```python
from build123d import *

# Parameters (mm, degrees)
SKETCH1_R                          = 14
BOSS_EXTRUDE1_DEPTH                = 20.5
SKETCH2_R                          = 12
CUT_EXTRUDE1_DEPTH                 = 17.5
CHAMFER1_SIZE                      = 1.5
SKETCH3_W                          = 0.15
SKETCH3_H                          = 0.25
SKETCH4_R                          = 4.45
BOSS_EXTRUDE2_DEPTH                = 1.5
BOSS_EXTRUDE2_DEPTH_BACK           = 4.5
SKETCH10_R                         = 4.45
BOSS_EXTRUDE3_DEPTH                = 3.5
BOSS_EXTRUDE3_TAPER                = 30
SKETCH5_R                          = 1.5
CUT_EXTRUDE2_DEPTH                 = 23
CUT_EXTRUDE3_DEPTH                 = 4.5
M1_6X0_35_TAPPED_HOLE1_D           = 1.25
M1_6X0_35_TAPPED_HOLE1_DEPTH       = 4.25
M1_6X0_35_TAPPED_HOLE1_TIP         = 0.375537887
M2_CLEARANCE_HOLE4_D               = 2.2
M2_CLEARANCE_HOLE4_DEPTH           = 3.5
M2_CLEARANCE_HOLE4_TIP             = 0.660946681
M2_CLEARANCE_HOLE4_ON_FACE_2_D     = 2.2
M2_CLEARANCE_HOLE4_ON_FACE_2_DEPTH = 3.5
M2_CLEARANCE_HOLE4_ON_FACE_2_TIP   = 0.660946681


with BuildPart() as part:
    # Sketch1 → Boss-Extrude1 (new body)
    with BuildSketch(Plane(origin=(0, 0, 0), x_dir=(1, 0, 0), z_dir=(0, 1, 0))):
        Circle(SKETCH1_R)
    extrude(amount=BOSS_EXTRUDE1_DEPTH)

    # Sketch2 → Cut-Extrude1 (cut)
    with BuildSketch(Plane.XZ):
        Circle(SKETCH2_R)
    extrude(amount=-CUT_EXTRUDE1_DEPTH, mode=Mode.SUBTRACT)

    # Chamfer1
    chamfer1_edges = [part.edges().sort_by_distance(p)[0] for p in [
        (-14, 20.5, 0),
    ]]
    chamfer(chamfer1_edges, length=CHAMFER1_SIZE)

    # Sketch3 → Cut-Revolve1 (revolve, cut)
    with BuildSketch(Plane(origin=(0, 0, 0), x_dir=(0, 0, -1), z_dir=(1, 0, 0))):
        with Locations((13.925, 14.875)):
            Rectangle(SKETCH3_W, SKETCH3_H)
    revolve(axis=Axis((0, 20.5, 0), (0, -1, 0)), mode=Mode.SUBTRACT)

    # Sketch4 → Boss-Extrude2 (add, two sides)
    with BuildSketch(Plane(origin=(0, 20.5, 0), x_dir=(1, 0, 0), z_dir=(0, 1, 0))) as boss_extrude2_sk:
        Circle(SKETCH4_R)
    extrude(amount=BOSS_EXTRUDE2_DEPTH)
    extrude(boss_extrude2_sk.sketch, amount=-BOSS_EXTRUDE2_DEPTH_BACK)

    # Sketch10 → Boss-Extrude3 (add)
    with BuildSketch(Plane.XZ.offset(-16)):
        Circle(SKETCH10_R)
    extrude(amount=BOSS_EXTRUDE3_DEPTH, taper=BOSS_EXTRUDE3_TAPER)

    # Sketch5 → Cut-Extrude2 (cut, through all)
    with BuildSketch(Plane(origin=(0, 22, 0), x_dir=(1, 0, 0), z_dir=(0, 1, 0))):
        Circle(SKETCH5_R)
    extrude(amount=-CUT_EXTRUDE2_DEPTH, mode=Mode.SUBTRACT)

    # Sketch6 → Cut-Extrude3 (cut)
    with BuildSketch(Plane(origin=(0, 20.5, 0), x_dir=(1, 0, 0), z_dir=(0, 1, 0))):
        with BuildLine():
            ThreePointArc((-10.0036, -7.495197598), (-4.6, 0), (-10.0036, 7.495197598))
            ThreePointArc((-10.0036, 7.495197598), (-12.5, 0), (-10.0036, -7.495197598))
        make_face()
        with BuildLine():
            ThreePointArc((-10.0036, 7.495197598), (-10.789488556, 7.712596878), (-11.5936, 7.847830212))
            ThreePointArc((-11.5936, 7.847830212), (-14, 0), (-11.5936, -7.847830212))
            ThreePointArc((-11.5936, -7.847830212), (-10.789488556, -7.712596878), (-10.0036, -7.495197598))
            ThreePointArc((-10.0036, -7.495197598), (-12.5, 0), (-10.0036, 7.495197598))
        make_face()
        with BuildLine():
            ThreePointArc((-9.006237245, -8.668199968), (-6.25, -10.825317547), (-3.003762755, -12.133730231))
            ThreePointArc((-3.003762755, -12.133730231), (-4.5, -7.794228634), (-9.006237245, -8.668199968))
        make_face()
        with BuildLine():
            ThreePointArc((-9.677498914, -10.116620719), (-7, -12.124355653), (-3.922501086, -13.439270264))
            ThreePointArc((-3.922501086, -13.439270264), (-3.387703302, -12.839581088), (-3.003762755, -12.133730231))
            ThreePointArc((-3.003762755, -12.133730231), (-6.25, -10.825317547), (-9.006237245, -8.668199968))
            ThreePointArc((-9.006237245, -8.668199968), (-9.425551745, -9.353627664), (-9.677498914, -10.116620719))
        make_face()
        with BuildLine():
            ThreePointArc((-0.999620328, -13.964267227), (7, -12.124355653), (12.593220328, -6.116437015))
            ThreePointArc((12.593220328, -6.116437015), (12.074049103, -5.487672744), (11.492831527, -4.91577293))
            ThreePointArc((11.492831527, -4.91577293), (6.25, -10.825317547), (-1.489231527, -12.410970529))
            ThreePointArc((-1.489231527, -12.410970529), (-1.284560547, -13.200269622), (-0.999620328, -13.964267227))
        make_face()
        with BuildLine():
            ThreePointArc((-1.489231527, -12.410970529), (6.25, -10.825317547), (11.492831527, -4.91577293))
            ThreePointArc((11.492831527, -4.91577293), (2.3, -3.983716857), (-1.489231527, -12.410970529))
        make_face()
        with BuildLine():
            ThreePointArc((12.5, 0), (12.376893794, 1.75), (12.01, 3.465530262))
            ThreePointArc((12.01, 3.465530262), (9, 0), (12.01, -3.465530262))
            ThreePointArc((12.01, -3.465530262), (12.376893794, -1.75), (12.5, 0))
        make_face()
        with BuildLine():
            ThreePointArc((13.6, -3.322649545), (13.899640283, -1.673320053), (14, 0))
            ThreePointArc((14, 0), (13.899640283, 1.673320053), (13.6, 3.322649545))
            ThreePointArc((13.6, 3.322649545), (12.813255048, 3.485953424), (12.01, 3.465530262))
            ThreePointArc((12.01, 3.465530262), (12.376893794, 1.75), (12.5, 0))
            ThreePointArc((12.5, 0), (12.376893794, -1.75), (12.01, -3.465530262))
            ThreePointArc((12.01, -3.465530262), (12.813255048, -3.485953424), (13.6, -3.322649545))
        make_face()
        with BuildLine():
            ThreePointArc((11.492831527, 4.91577293), (12.074049103, 5.487672744), (12.593220328, 6.116437015))
            ThreePointArc((12.593220328, 6.116437015), (7, 12.124355653), (-0.999620328, 13.964267227))
            ThreePointArc((-0.999620328, 13.964267227), (-1.284560547, 13.200269622), (-1.489231527, 12.410970529))
            ThreePointArc((-1.489231527, 12.410970529), (6.25, 10.825317547), (11.492831527, 4.91577293))
        make_face()
        with BuildLine():
            ThreePointArc((-1.489231527, 12.410970529), (2.3, 3.983716857), (11.492831527, 4.91577293))
            ThreePointArc((11.492831527, 4.91577293), (6.25, 10.825317547), (-1.489231527, 12.410970529))
        make_face()
        with BuildLine():
            ThreePointArc((-9.006237245, 8.668199968), (-4.5, 7.794228634), (-3.003762755, 12.133730231))
            ThreePointArc((-3.003762755, 12.133730231), (-6.25, 10.825317547), (-9.006237245, 8.668199968))
        make_face()
        with BuildLine():
            ThreePointArc((-3.003762755, 12.133730231), (-3.387703302, 12.839581088), (-3.922501086, 13.439270264))
            ThreePointArc((-3.922501086, 13.439270264), (-7, 12.124355653), (-9.677498914, 10.116620719))
            ThreePointArc((-9.677498914, 10.116620719), (-9.425551745, 9.353627664), (-9.006237245, 8.668199968))
            ThreePointArc((-9.006237245, 8.668199968), (-6.25, 10.825317547), (-3.003762755, 12.133730231))
        make_face()
    extrude(amount=-CUT_EXTRUDE3_DEPTH, mode=Mode.SUBTRACT)

    # M1.6x0.35 Tapped Hole1
    with Locations(Plane(origin=(6, 20.5, 0), x_dir=(0, 0, 1), z_dir=(0, 1, 0))):
        with Locations((0, 0), (5.196152423, -9), (-5.196152423, -9)):
            Hole(M1_6X0_35_TAPPED_HOLE1_D / 2, depth=M1_6X0_35_TAPPED_HOLE1_DEPTH)
            with Locations((0, 0, -(M1_6X0_35_TAPPED_HOLE1_DEPTH + M1_6X0_35_TAPPED_HOLE1_TIP / 2))):  # 118° drill point
                Cone(0, M1_6X0_35_TAPPED_HOLE1_D / 2, M1_6X0_35_TAPPED_HOLE1_TIP, mode=Mode.SUBTRACT)

    # M2 Clearance Hole4
    with Locations(Plane(origin=(-4.6, 18.5, 0), x_dir=(0, 0, -1), z_dir=(-1, 0, 0))):
        with Locations((0, 0)):
            Hole(M2_CLEARANCE_HOLE4_D / 2, depth=M2_CLEARANCE_HOLE4_DEPTH)
            with Locations((0, 0, -(M2_CLEARANCE_HOLE4_DEPTH + M2_CLEARANCE_HOLE4_TIP / 2))):  # 118° drill point
                Cone(0, M2_CLEARANCE_HOLE4_D / 2, M2_CLEARANCE_HOLE4_TIP, mode=Mode.SUBTRACT)

    # M2 Clearance Hole4 on face 2
    with Locations(Plane(origin=(2.3, 18.5, 3.983716857), x_dir=(0.866025303, 0, -0.500000175), z_dir=(0.500000175, 0, 0.866025303))):
        with Locations((0, 0)):
            Hole(M2_CLEARANCE_HOLE4_ON_FACE_2_D / 2, depth=M2_CLEARANCE_HOLE4_ON_FACE_2_DEPTH)
            with Locations((0, 0, -(M2_CLEARANCE_HOLE4_ON_FACE_2_DEPTH + M2_CLEARANCE_HOLE4_ON_FACE_2_TIP / 2))):  # 118° drill point
                Cone(0, M2_CLEARANCE_HOLE4_ON_FACE_2_D / 2, M2_CLEARANCE_HOLE4_ON_FACE_2_TIP, mode=Mode.SUBTRACT)


solid = part.part
```
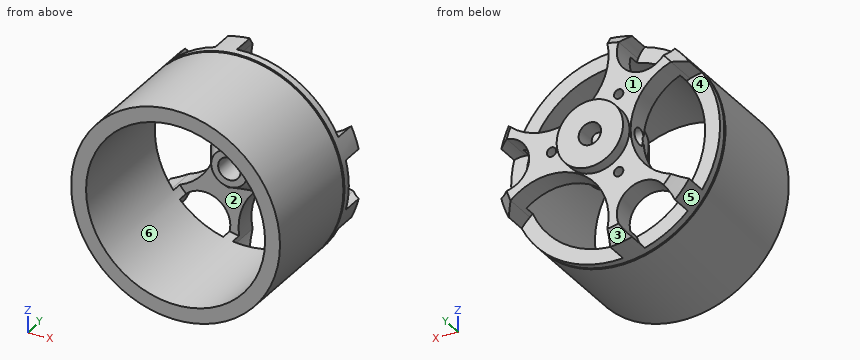
Verification items for the finished model (mm, model axes). Face numbers are marked on the shaded views. A direction names the side the tool comes from. Round coordinates to 2 decimals unless told otherwise and drop trailing zeros. Order: outer loops, then holes, each group sorted by start corner. A loop starts at its lowest first (then second) coordinate and runs counter-clockwise, first axis right, second up. Notation, with made-up numbers: (-17, 80) -> (9, 80) arc R24 cw to (9, 102) -> close; hole circle Ø5 at (2, 14). An arc over 180 degrees is marked (long way). Put each result on its own line as item: value. Start each with the question number.
(1) Section check D-D (y = 18.5). State how many separate pieces and enclosed holes the cut face has, then the cut area to 3 significant figures.
(2) Material ranges on line 1 along X through (y, z) = (18.5, 0) (3 decimals); line 2 along Z through (x, y) = (0, 8.5); line 3 along X through (y, z) = (17.25, 0), recorded low to high.
(3) Depth check by flat-ended pin: pin 1 Ø2 at (x, z) = (-3, -5.2) entering from +Y; pin 2 Ø8 at (x, z) = (-0.5, -0.5) entering from -Y; pin 3 Ø1.5 at (x, z) = (-8.5, 8) entering from -Y; pin 4 Ø8 at (y, z) = (5.5, 10.5) entering from -X. Enter the tip coordinate at first touch or a pass-through.
(4) Tool access check on the marked faces 4, 5 and 6. Record the directions out of +Z, -Z, +X, -X, +Y, -Y that give a thin tool (end or side, any length) a straight path to the whole face; none if there is none.
(5) Section check B-B (x = 10.5). Enter the section's corners in (y, z).
(6) Section check A-A (z = 11.25). Enter the section's corners in (x, y), then the cut area to 3 significant figures.
(7) Section check C-C (y = 4). Enter the section's corners in (x, z), then the cut area to 3 significant figures.
(8) Draft check along Z on the marked faces 1, 2 and 3. Enter one of: +Z half, -Z half, draft (parallel to the pull), parting line (faces both ways), or undercut.
Completed:
1. separate pieces: 2
1. enclosed holes: 3
1. area: 177 mm2
2. line 1: x = 1.5 to 5.375, 6.625 to 9
2. line 2: z = -14 to -12, 12 to 14
2. line 3: x = -4.45 to -1.5, 1.5 to 4.45
3. pin 1: stops at y = 20.5
3. pin 2: stops at y = 12.5
3. pin 3: stops at y = 0
3. pin 4: stops at x = -12.4
4. face 4: -X, +Y
4. face 5: +Y, -Y
4. face 6: -Y
5. outline: (0, -9.26) -> (14.75, -9.26) -> (14.75, -9.03) -> (15, -9.03) -> (15, -9.26) -> (16, -9.26) -> (16, -5.81) -> (0, -5.81) -> close; (0, 5.81) -> (16, 5.81) -> (16, 9.26) -> (15, 9.26) -> (15, 9.03) -> (14.75, 9.03) -> (14.75, 9.26) -> (0, 9.26) -> close; (17.5, -4.17) -> (20.5, -4.17) -> (20.5, -2.87) -> (17.5, -2.87) -> close; (17.5, 2.87) -> (20.5, 2.87) -> (20.5, 4.17) -> (17.5, 4.17) -> close
6. outline: (-8.33, 0) -> (-4.18, 0) -> (-4.18, 16) -> (-8.33, 16) -> (-8.33, 15) -> (-8.08, 15) -> (-8.08, 14.75) -> (-8.33, 14.75) -> close; (-2.78, 17.5) -> (-1.64, 17.5) -> (-1.64, 20.5) -> (-2.78, 20.5) -> close; (4.18, 0) -> (8.33, 0) -> (8.33, 14.75) -> (8.08, 14.75) -> (8.08, 15) -> (8.33, 15) -> (8.33, 16) -> (4.18, 16) -> close
6. area: 136 mm2
7. outline: circle Ø28 at (0, 0); hole circle Ø24 at (0, 0)
7. area: 163 mm2
8. face 1: draft
8. face 2: undercut
8. face 3: -Z half
